The listing builds one solid part. Answer for the finished solid, in the listing's coordinates (mm). A direction names the side the tool comes from. Give positions to 0.01 mm unless a question says otherwise; leave off trailing zeros. Use one line per item in the form item = value. Start each with the question number.
1. Straight lines are drawn through the part: line 1 (Z direction, x = 56, y = 0.7) (3 decimals); line 2 (Y direction, x = 29.5, z = 1.5); line 3 (Z direction, x = 17.5, y = 5.75). For each, find the intervals that lie inside material, in ascending order. Write a range as from..to.
2. The part is cut by section A-A (y = 1.75). Give the number of separate pieces and of enclosed holes in the cut face, and give its area (3 significant figures).
3. For faces 4 (the face through (35.1, 6.9, -0.4)), 5 (the face through (58.98, 0.62, 0.94)), 6 (the face through (-3.62, 0.12, 0.08)), determine the directions among +Z, -Z, +X, -X, +Y, -Y from which every point of the face is accessible in a straight line to the end or side of a thin tool.
4. The mould has two halves that part along Z. Classify faces 1 (the face through (19.1, 6.9, -0.4)), 2 (the face through (4, 0, 0)), 3 (the face through (32, 4, 3.9)): released by +Z, released by -Z, zero draft, split by the parting line, or undercut.
5. Each of these flat-tipped pins is pushed along its axis until it touches: pin 1 Ø3 at (x, z) = (57.5, -0.5) entering from -Y; pin 2 Ø4.5 at (x, z) = (32, 0) entering from -Y. Where does it stop, or does it pass through?
from build123d import *

# Parameters (mm, degrees)
BOSS_EXTRUDE1_DEPTH       = 7.3
SKETCH2_R                 = 2.475
CUT_EXTRUDE1_DEPTH        = 69.402558432
SKETCH3_R                 = 3.125
CUT_EXTRUDE2_DEPTH        = 0.85
LPATTERN1_COUNT           = 9
LPATTERN1_PITCH           = 8
LPATTERN1_COPY_1_SKETCH_R = 3.125
LPATTERN1_COPY_1_DEPTH    = 0.85
LPATTERN1_COPY_2_SKETCH_R = 3.125
LPATTERN1_COPY_2_DEPTH    = 0.85
LPATTERN1_COPY_3_SKETCH_R = 3.125
LPATTERN1_COPY_3_DEPTH    = 0.85
LPATTERN1_COPY_4_SKETCH_R = 3.125
LPATTERN1_COPY_4_DEPTH    = 0.85
LPATTERN1_COPY_5_SKETCH_R = 3.125
LPATTERN1_COPY_5_DEPTH    = 0.85
LPATTERN1_COPY_6_SKETCH_R = 3.125
LPATTERN1_COPY_6_DEPTH    = 0.85
LPATTERN1_COPY_7_SKETCH_R = 3.125
LPATTERN1_COPY_7_DEPTH    = 0.85
LPATTERN1_COPY_8_SKETCH_R = 3.125
LPATTERN1_COPY_8_DEPTH    = 0.85
CHAMFER1_SIZE             = 0.4


with BuildPart() as part:
    # Sketch1 → Boss-Extrude1 (new body)
    with BuildSketch(Plane(origin=(0, 0, 0), x_dir=(1, 0, 0), z_dir=(0, 1, 0))):
        with BuildLine():
            Line((0, 3.9), (64, 3.9))
            ThreePointArc((64, 3.9), (67.9, 0), (64, -3.9))
            Line((64, -3.9), (0, -3.9))
            ThreePointArc((0, -3.9), (-3.9, 0), (0, 3.9))
        make_face()
    extrude(amount=BOSS_EXTRUDE1_DEPTH)

    # Sketch2 → Cut-Extrude1 (cut, through all)
    with BuildSketch(Plane(origin=(0, 7.3, 0), x_dir=(1, 0, 0), z_dir=(0, 1, 0))):
        with Locations(Location((0, 0, 0), (0, 0, 270))):
            Circle(SKETCH2_R)
    cut_extrude1 = extrude(amount=-CUT_EXTRUDE1_DEPTH, mode=Mode.SUBTRACT)

    # Sketch3 → Cut-Extrude2 (cut)
    with BuildSketch(Plane(origin=(0, 7.3, 0), x_dir=(1, 0, 0), z_dir=(0, 1, 0))):
        with Locations(Location((0, 0, 0), (0, 0, 270))):
            Circle(SKETCH3_R)
    cut_extrude2 = extrude(amount=-CUT_EXTRUDE2_DEPTH, mode=Mode.SUBTRACT)

    # Mirror1: Cut-Extrude2 across plane
    add(cut_extrude2.mirror(Plane.ZX.offset(3.65)), mode=Mode.SUBTRACT)

    # LPattern1: Cut-Extrude1, Cut-Extrude2 ×9
    with Locations(*[(i * LPATTERN1_PITCH, 0, 0) for i in range(1, LPATTERN1_COUNT)]):
        add(cut_extrude1, mode=Mode.SUBTRACT)
        add(cut_extrude2, mode=Mode.SUBTRACT)

    # LPattern1 copy 1 sketch → LPattern1 copy 1 (cut)
    with BuildSketch(Plane(origin=(8, 0, 0), x_dir=(1, 0, 0), z_dir=(0, -1, 0))):
        Circle(LPATTERN1_COPY_1_SKETCH_R)
    extrude(amount=-LPATTERN1_COPY_1_DEPTH, mode=Mode.SUBTRACT)

    # LPattern1 copy 2 sketch → LPattern1 copy 2 (cut)
    with BuildSketch(Plane(origin=(16, 0, 0), x_dir=(1, 0, 0), z_dir=(0, -1, 0))):
        Circle(LPATTERN1_COPY_2_SKETCH_R)
    extrude(amount=-LPATTERN1_COPY_2_DEPTH, mode=Mode.SUBTRACT)

    # LPattern1 copy 3 sketch → LPattern1 copy 3 (cut)
    with BuildSketch(Plane(origin=(24, 0, 0), x_dir=(1, 0, 0), z_dir=(0, -1, 0))):
        Circle(LPATTERN1_COPY_3_SKETCH_R)
    extrude(amount=-LPATTERN1_COPY_3_DEPTH, mode=Mode.SUBTRACT)

    # LPattern1 copy 4 sketch → LPattern1 copy 4 (cut)
    with BuildSketch(Plane(origin=(32, 0, 0), x_dir=(1, 0, 0), z_dir=(0, -1, 0))):
        Circle(LPATTERN1_COPY_4_SKETCH_R)
    extrude(amount=-LPATTERN1_COPY_4_DEPTH, mode=Mode.SUBTRACT)

    # LPattern1 copy 5 sketch → LPattern1 copy 5 (cut)
    with BuildSketch(Plane(origin=(40, 0, 0), x_dir=(1, 0, 0), z_dir=(0, -1, 0))):
        Circle(LPATTERN1_COPY_5_SKETCH_R)
    extrude(amount=-LPATTERN1_COPY_5_DEPTH, mode=Mode.SUBTRACT)

    # LPattern1 copy 6 sketch → LPattern1 copy 6 (cut)
    with BuildSketch(Plane(origin=(48, 0, 0), x_dir=(1, 0, 0), z_dir=(0, -1, 0))):
        Circle(LPATTERN1_COPY_6_SKETCH_R)
    extrude(amount=-LPATTERN1_COPY_6_DEPTH, mode=Mode.SUBTRACT)

    # LPattern1 copy 7 sketch → LPattern1 copy 7 (cut)
    with BuildSketch(Plane(origin=(56, 0, 0), x_dir=(1, 0, 0), z_dir=(0, -1, 0))):
        Circle(LPATTERN1_COPY_7_SKETCH_R)
    extrude(amount=-LPATTERN1_COPY_7_DEPTH, mode=Mode.SUBTRACT)

    # LPattern1 copy 8 sketch → LPattern1 copy 8 (cut)
    with BuildSketch(Plane(origin=(64, 0, 0), x_dir=(1, 0, 0), z_dir=(0, -1, 0))):
        Circle(LPATTERN1_COPY_8_SKETCH_R)
    extrude(amount=-LPATTERN1_COPY_8_DEPTH, mode=Mode.SUBTRACT)

    # Chamfer1
    # the kernel refuses this chamfer: 0.4 mm, written as the material it takes off along each edge
    with BuildSketch(Plane(origin=(8, 0, 0), x_dir=(1, 0, 0), z_dir=(0, 0, -1))) as chamfer1_piece_1:
        Polygon((3.125 + CHAMFER1_SIZE, 0), (3.125, -CHAMFER1_SIZE), (3.125, 0), align=None)
    revolve(axis=Axis((8, 0, 0), (0, -1, 0)), mode=Mode.SUBTRACT)
    with BuildSketch(Plane(origin=(16, 0, 0), x_dir=(1, 0, 0), z_dir=(0, 0, -1))) as chamfer1_piece_2:
        Polygon((3.125 + CHAMFER1_SIZE, 0), (3.125, -CHAMFER1_SIZE), (3.125, 0), align=None)
    revolve(axis=Axis((16, 0, 0), (0, -1, 0)), mode=Mode.SUBTRACT)
    with BuildSketch(Plane(origin=(24, 0, 0), x_dir=(1, 0, 0), z_dir=(0, 0, -1))) as chamfer1_piece_3:
        Polygon((3.125 + CHAMFER1_SIZE, 0), (3.125, -CHAMFER1_SIZE), (3.125, 0), align=None)
    revolve(axis=Axis((24, 0, 0), (0, -1, 0)), mode=Mode.SUBTRACT)
    with BuildSketch(Plane(origin=(32, 0, 0), x_dir=(1, 0, 0), z_dir=(0, 0, -1))) as chamfer1_piece_4:
        Polygon((3.125 + CHAMFER1_SIZE, 0), (3.125, -CHAMFER1_SIZE), (3.125, 0), align=None)
    revolve(axis=Axis((32, 0, 0), (0, -1, 0)), mode=Mode.SUBTRACT)
    with BuildSketch(Plane(origin=(40, 0, 0), x_dir=(1, 0, 0), z_dir=(0, 0, -1))) as chamfer1_piece_5:
        Polygon((3.125 + CHAMFER1_SIZE, 0), (3.125, -CHAMFER1_SIZE), (3.125, 0), align=None)
    revolve(axis=Axis((40, 0, 0), (0, -1, 0)), mode=Mode.SUBTRACT)
    with BuildSketch(Plane(origin=(48, 0, 0), x_dir=(1, 0, 0), z_dir=(0, 0, -1))) as chamfer1_piece_6:
        Polygon((3.125 + CHAMFER1_SIZE, 0), (3.125, -CHAMFER1_SIZE), (3.125, 0), align=None)
    revolve(axis=Axis((48, 0, 0), (0, -1, 0)), mode=Mode.SUBTRACT)
    with BuildSketch(Plane(origin=(56, 0, 0), x_dir=(1, 0, 0), z_dir=(0, 0, -1))) as chamfer1_piece_7:
        Polygon((3.125 + CHAMFER1_SIZE, 0), (3.125, -CHAMFER1_SIZE), (3.125, 0), align=None)
    revolve(axis=Axis((56, 0, 0), (0, -1, 0)), mode=Mode.SUBTRACT)
    with BuildSketch(Plane(origin=(64, 0, 0), x_dir=(1, 0, 0), z_dir=(0, 0, -1))) as chamfer1_piece_8:
        Polygon((3.125 + CHAMFER1_SIZE, 0), (3.125, -CHAMFER1_SIZE), (3.125, 0), align=None)
    revolve(axis=Axis((64, 0, 0), (0, -1, 0)), mode=Mode.SUBTRACT)
    with BuildSketch(Plane(origin=(0, 0, 0), x_dir=(0, 0, 1), z_dir=(-1, 0, 0))) as chamfer1_piece_9:
        Polygon((3.125 + CHAMFER1_SIZE, 0), (3.125, CHAMFER1_SIZE), (3.125, 0), align=None)
    revolve(axis=Axis((0, 0, 0), (0, 1, 0)), mode=Mode.SUBTRACT)
    with BuildSketch(Plane(origin=(0, 0, -3.9), x_dir=(0, -0.027495876610586386, 0.9996219169112968), z_dir=(1, 0, 0))) as chamfer1_piece_10:
        Polygon((CHAMFER1_SIZE * 0.999621916911, -CHAMFER1_SIZE * 0.0274958766106), (-CHAMFER1_SIZE * 0.0274958766106, -CHAMFER1_SIZE * 0.999621916911), (0, 0), align=None)
    extrude(amount=64, mode=Mode.SUBTRACT)
    with BuildSketch(Plane(origin=(64, 0, 0), x_dir=(0, 0, -1), z_dir=(-1, 0, 0))) as chamfer1_piece_11:
        Polygon((3.9, -CHAMFER1_SIZE), (3.9 - CHAMFER1_SIZE, 0), (3.9, 0), align=None)
    revolve(axis=Axis((64, 0, 0), (0, -1, 0)), revolution_arc=180, mode=Mode.SUBTRACT)
    with BuildSketch(Plane(origin=(64, 0, 3.9), x_dir=(0, 0.9996219169112968, 0.027495876610586275), z_dir=(-1, 0, 0))) as chamfer1_piece_12:
        Polygon((CHAMFER1_SIZE * 0.999621916911, CHAMFER1_SIZE * 0.0274958766106), (-CHAMFER1_SIZE * 0.0274958766106, CHAMFER1_SIZE * 0.999621916911), (0, 0), align=None)
    extrude(amount=64, mode=Mode.SUBTRACT)
    with BuildSketch(Plane(origin=(0, 0, 0), x_dir=(0, 0, 1), z_dir=(1, 0, 0))) as chamfer1_piece_13:
        Polygon((3.9, -CHAMFER1_SIZE), (3.9 - CHAMFER1_SIZE, 0), (3.9, 0), align=None)
    revolve(axis=Axis((0, 0, 0), (0, -1, 0)), revolution_arc=180, mode=Mode.SUBTRACT)


solid = part.part
Derived:
q1.line_1 = -3.9..-3.125, 3.125..3.9
q1.line_2 = 0.85..6.45
q1.line_3 = -3.9..-1.97, 1.97..3.9
q2.separate_pieces = 1
q2.enclosed_holes = 9
q2.area = 374 mm2
q3.face_4 = +Y
q3.face_5 = -Y
q3.face_6 = -X, -Y
q4.face_1 = undercut
q4.face_2 = zero draft
q4.face_3 = released by +Z
q5.pin_1 = 0.85
q5.pin_2 = through
